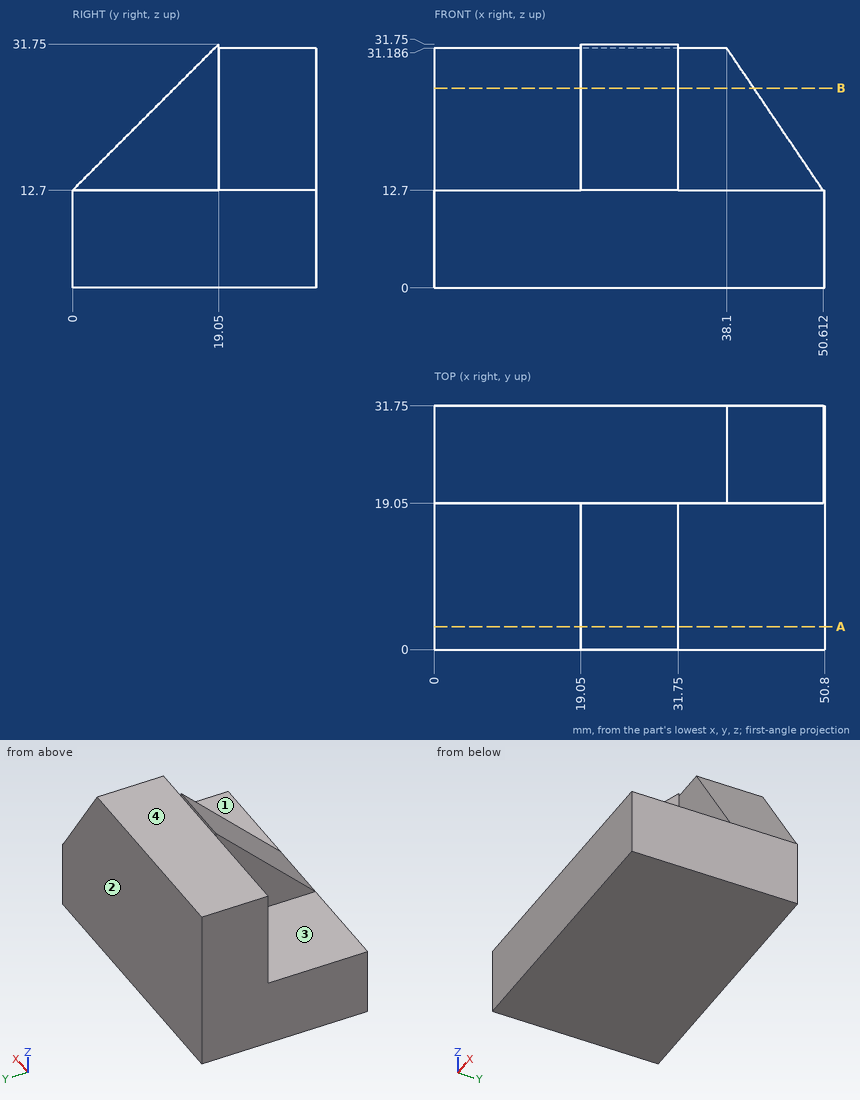
Design review of the part shown in the three views and the two pictorial views. Dimensions are in mm from the part's minimum x, y and z. A direction names the side the tool comes from. Round coordinates to 2 decimals unless told otherwise and drop trailing zeros. Write each loop counter-clockwise with the first axis right and the second up, starting at its lowest first coordinate (ties: lowest second). Pieces come first, ordered by that corner, then holes. Notation, with made-up numbers: (-2, 5) -> (51, 5) arc R28 cw to (51, 35) -> close; hole circle Ø4 at (-3, -28). An arc over 180 degrees is marked (long way). Use one line per item in the form item = value.
1) Clearance check with flat-ended pins moving along their axes: pin 1 (9.5 mm diameter, centred on x = 39, y = 9, fed in from +Z); pin 2 (8 mm diameter, centred on y = 23.5, z = 21.5, fed in from +X); pin 3 (5.5 mm diameter, centred on x = 44, z = 26, fed in from -Y). State where each tip first meets the part, or that it passes through.
Found:
pin_1 = 12.7
pin_2 = 47.36
pin_3 = 19.05
2) To check wall thickness, follow L1, parallel to Y at x = 8, z = 29; L2, parallel to Z at x = 12.5, y = 5.5; L3, parallel to Z at x = 12.5, y = 21 (1 decimal). State the ranges of each line that lie inside material, in increasing order. Write a range as from..to.
Found:
L1 = 19.05..31.75
L2 = 0..12.7
L3 = 0..31.2
3) Take a section at A-A, the plane y = 3. Write out the cut boundary in (x, z).
Found:
outline = (0, 0) -> (50.8, 0) -> (50.8, 12.7) -> (31.75, 12.7) -> (31.75, 15.7) -> (19.05, 15.7) -> (19.05, 12.7) -> (0, 12.7) -> close
4) Tool access review of the marked faces 1, 2, 3 and 4: name each direction out of +Z, -Z, +X, -X, +Y, -Y from which nothing blocks a thin tool from reaching the whole face with its end or side.
Found:
face_1 = +Z, +X, -Y
face_2 = +Z, -Z, +X, -X, +Y
face_3 = +Z, -X, -Y
face_4 = +Z, +X, -X, +Y
5) Take a section at B-B, the plane z = 26. Write out the cut boundary in (x, y).
Found:
outline = (0, 19.05) -> (19.05, 19.05) -> (19.05, 13.3) -> (31.75, 13.3) -> (31.75, 19.05) -> (41.61, 19.05) -> (41.61, 31.75) -> (0, 31.75) -> close
